Build history of the part. All positions in model axes, mm. Face numbers are marked on the shaded views. A direction names the side the tool comes from. Give positions to 0.01 mm unless a question says otherwise; leave off trailing zeros. Loops run counter-clockwise (first coordinate to the right, second up) from the corner with the lowest first, then second, coordinate; pieces in that order, holes last. Notation, with made-up numbers: (-3.75, 1) -> (44.25, 1) arc R29 ccw to (44.25, 38) -> close; hole circle Ø2 at (-12.5, 61.5). An arc over 180 degrees is marked (long way). Answer as a JSON object with one key per item and string values. Group by question number.
from build123d import *

# Parameters (mm, degrees)
SKETCH1_R               = 15.5
BOSS_EXTRUDE1_DEPTH     = 5
SKETCH2_R               = 15.5
BOSS_EXTRUDE2_DEPTH     = 15
CUT_EXTRUDE7_DEPTH      = 20.5
CUT_EXTRUDE7_DEPTH_BACK = 26
SKETCH18_R              = 1.6
CUT_EXTRUDE8_DEPTH      = 6
SKETCH19_R              = 2.05
CUT_EXTRUDE9_DEPTH      = 6
CUT_EXTRUDE10_REACH     = 4
SKETCH20_R              = 4


with BuildPart() as part:
    # Sketch1 → Boss-Extrude1 (new body)
    with BuildSketch(Plane(origin=(0, 0, 0), x_dir=(1, 0, 0), z_dir=(0, 1, 0))):
        Circle(SKETCH1_R)
    extrude(amount=BOSS_EXTRUDE1_DEPTH)

    # Sketch2 → Boss-Extrude2 (add)
    with BuildSketch(Plane.XZ):
        with BuildLine():
            Line((-22, -25), (4.323483194, -19.014665211))
            ThreePointArc((4.323483194, -19.014665211), (18.889988887, 4.839247858), (-5.351429285, 18.751325409))
            Line((-5.351429285, 18.751325409), (-22, 14))
            Line((-22, 14), (-22, -25))
        make_face()
        Circle(SKETCH2_R, mode=Mode.SUBTRACT)
    extrude(amount=-BOSS_EXTRUDE2_DEPTH)

    # Sketch17 → Cut-Extrude7 (cut, two sides)
    with BuildSketch(Plane.XY) as cut_extrude7_sk:
        Polygon((19.5, 0), (-14, 0), (19.5, 3), align=None)
    extrude(amount=CUT_EXTRUDE7_DEPTH, mode=Mode.SUBTRACT)
    extrude(cut_extrude7_sk.sketch, amount=-CUT_EXTRUDE7_DEPTH_BACK, mode=Mode.SUBTRACT)

    # Sketch18 → Cut-Extrude8 (cut, through all)
    with BuildSketch(Plane(origin=(0, 5, 0), x_dir=(1, 0, 0), z_dir=(0, 1, 0))):
        Circle(SKETCH18_R)
    extrude(amount=-CUT_EXTRUDE8_DEPTH, mode=Mode.SUBTRACT)

    # Sketch19 → Cut-Extrude9 (cut)
    with BuildSketch(Plane.XZ):
        with Locations((-18, -5.5)):
            Circle(SKETCH19_R)
    extrude(amount=-CUT_EXTRUDE9_DEPTH, mode=Mode.SUBTRACT)

    # Sketch20 → Cut-Extrude10 (cut, up to next)
    with BuildSketch(Plane(origin=(0, 2, 0), x_dir=(1, 0, 0), z_dir=(0, 1, 0)), mode=Mode.PRIVATE) as cut_extrude10_sk1:
        Circle(SKETCH20_R)
    cut_extrude10_tool1 = extrude(cut_extrude10_sk1.sketch, amount=-CUT_EXTRUDE10_REACH, mode=Mode.PRIVATE) & part.part
    add(cut_extrude10_tool1.solids().sort_by_distance((0, 2, 0))[0], mode=Mode.SUBTRACT)


solid = part.part
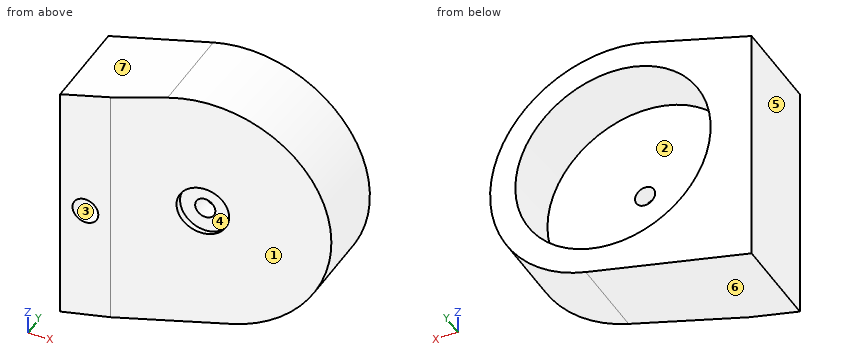
(1) Pull direction Z, two halves, no side cores. Call the marked faces 4, 5, 6 and 7: pulls with the +Z half, pulls with the -Z half, needs draft (parallel to the pull), parting line crosses it, or undercut.
(2) Saw through at C-C on y = 9. List the corners of the cut face in (x, z).
(3) 3-axis set-ups, long thin cutter, end or side, ignore diameter. For the marked faces 1, 2 and 3: which of +Z, -Z, +X, -X, +Y, -Y reach the whole face in a straight line?
(4) Saw through at D-D on x = -18. List the corners of the cut face in (y, z).
(5) Probe line 1 along X through (y, z) = (3.1, 0); line 2 along Y through (x, z) = (4, 5.5); line 3 along X through (y, z) = (6.5, 9.5). List the from-to ranges inside material, lowest first. Write a range as [from, to].
(6) Pin check, flat tips, straight feed: pin 1 (3.5 mm diameter, centred on x = 0, z = 0, fed in from -Y); pin 2 (6 mm diameter, centred on y = 9.5, z = 4, fed in from +X); pin 3 (1 mm diameter, centred on x = 11.5, z = -15.5, fed in from -Y). Stop position of each tip, or through.
(7) Saw through at B-B on x = 0. List the corners of the cut face in (y, z).
(8) Saw through at A-A on z = 0. List the corners of the cut face in (x, y).
Calculated:
{
 "1": {"face 4": "undercut", "face 5": "needs draft", "face 6": "pulls with the -Z half", "face 7": "pulls with the +Z half"},
 "2": {"outline": "(-22, -25) -> (4.32, -19.01) arc R19.5 ccw (long way) to (-5.35, 18.75) -> (-22, 14) -> close; hole circle Ø31 at (0, 0)"},
 "3": {"face 1": "+Z, -Z, +X, -Y", "face 2": "+Y", "face 3": "-Y"},
 "4": {"outline": "(0, -24.09) -> (15, -24.09) -> (15, 15.14) -> (0, 15.14) -> (0, -3.45) -> (6, -3.45) -> (6, -7.55) -> (0, -7.55) -> close"},
 "5": {"line 1": "x = [-22, -1.6], [1.6, 19.5]", "line 2": "y = [1.61, 5]", "line 3": "x = [-22, -12.25], [12.25, 17.03]"},
 "6": {"pin 1": "stops at y = 2", "pin 2": "stops at x = 19.47", "pin 3": "stops at y = 2.24"},
 "7": {"outline": "(1.25, -20) -> (15, -20) -> (15, -15.5) -> (5, -15.5) -> (5, -1.6) -> (2, -1.6) -> (2, -4) -> (1.25, -4) -> close; (1.25, 4) -> (2, 4) -> (2, 1.6) -> (5, 1.6) -> (5, 15.5) -> (15, 15.5) -> (15, 19.5) -> (1.25, 19.5) -> close"},
 "8": {"outline": "(-22, 0) -> (-14, 0) -> (-4, 0.9) -> (-4, 2) -> (-1.6, 2) -> (-1.6, 5) -> (-15.5, 5) -> (-15.5, 15) -> (-22, 15) -> close; (1.6, 2) -> (4, 2) -> (4, 1.61) -> (19.5, 3) -> (19.5, 15) -> (15.5, 15) -> (15.5, 5) -> (1.6, 5) -> close"}
}
